Check sheet for the modelled part. Datum: model origin and axes. Units: mm. A direction names the side the tool comes from. Round coordinates to 2 decimals unless told otherwise and drop trailing zeros. Write each loop counter-clockwise with the first axis right and the second up, starting at its lowest first coordinate (ties: lowest second). Pieces come first, ordered by that corner, then holes. Notation, with made-up numbers: (-14.75, -33) -> (43.25, -33) arc R12 cw to (43.25, -14) -> close; hole circle Ø7 at (36, -4). An arc over 180 degrees is marked (long way). Write item = value, one per line.
from build123d import *

# Parameters (mm, degrees)
SKETCH_1_W               = 42
SKETCH_1_H               = 42
SKETCH_1_R               = 1.85
EXTRUDE_1_DEPTH          = 5
FILLET_2_R               = 2
FILLET_3_R               = 2
FILLET_4_R               = 2
FILLET_5_R               = 2
CUT_EXTRUDE_3_DEPTH      = 31.116440693
SKETCH_6_W               = 14
SKETCH_6_H               = 11
CUT_EXTRUDE_4_DEPTH      = 31.116440693
SKETCH_8_R               = 1
CUT_EXTRUDE_6_DEPTH      = 31.116440693
SKETCH_9_R               = 3
CUT_EXTRUDE_7_DEPTH      = 2.7
SKETCH_11_W              = 27.9
SKETCH_11_H              = 28.4
CUT_EXTRUDE_14_DEPTH     = 2.7
CUT_EXTRUDE_15_DEPTH     = 1.5
HOLE_WIZARD_1_AT_2_COUNT = 2
HOLE_WIZARD_1_AT_2_PITCH = 31
HOLE_WIZARD_1_AT_3_COUNT = 2
HOLE_WIZARD_1_AT_3_PITCH = 43.840620434
HOLE_WIZARD_1_AT_4_COUNT = 2
HOLE_WIZARD_1_AT_4_PITCH = 31


with BuildPart() as part:
    # 草图1 → 凸台-拉伸1 (new body)
    with BuildSketch(Plane(origin=(0, 0, 0), x_dir=(1, 0, 0), z_dir=(0, 1, 0))):
        Rectangle(SKETCH_1_W, SKETCH_1_H)
        with Locations(Location((15.5, 15.5, 0), (0, 0, 270))):
            Circle(SKETCH_1_R, mode=Mode.SUBTRACT)
        with Locations(Location((-15.5, 15.5, 0), (0, 0, 270))):
            Circle(SKETCH_1_R, mode=Mode.SUBTRACT)
        with Locations(Location((-15.5, -15.5, 0), (0, 0, 270))):
            Circle(SKETCH_1_R, mode=Mode.SUBTRACT)
        with Locations(Location((15.5, -15.5, 0), (0, 0, 270))):
            Circle(SKETCH_1_R, mode=Mode.SUBTRACT)
    extrude(amount=EXTRUDE_1_DEPTH)

    # 圆角2
    fillet_2_edges = [part.edges().sort_by_distance(p)[0] for p in [
        (-21, 2.5, -21),
    ]]
    fillet(fillet_2_edges, radius=FILLET_2_R)

    # 圆角3
    fillet_3_edges = [part.edges().sort_by_distance(p)[0] for p in [
        (-21, 2.5, 21),
    ]]
    fillet(fillet_3_edges, radius=FILLET_3_R)

    # 圆角4
    fillet_4_edges = [part.edges().sort_by_distance(p)[0] for p in [
        (21, 2.5, 21),
    ]]
    fillet(fillet_4_edges, radius=FILLET_4_R)

    # 圆角5
    fillet_5_edges = [part.edges().sort_by_distance(p)[0] for p in [
        (21, 2.5, -21),
    ]]
    fillet(fillet_5_edges, radius=FILLET_5_R)

    # 草图5 → 切除-拉伸3 (cut, through all)
    with BuildSketch(Plane.XZ):
        Polygon((-15.5, -21), (-10, -15.5), (10, -15.5), (15.5, -21), align=None)
    extrude(amount=-CUT_EXTRUDE_3_DEPTH, mode=Mode.SUBTRACT)

    # 草图6 → 切除-拉伸4 (cut, through all)
    with BuildSketch(Plane.XZ):
        with Locations((-3, 15.5)):
            Rectangle(SKETCH_6_W, SKETCH_6_H)
    extrude(amount=-CUT_EXTRUDE_4_DEPTH, mode=Mode.SUBTRACT)

    # 草图8 → 切除-拉伸6 (cut, through all)
    with BuildSketch(Plane(origin=(0, 5, 0), x_dir=(1, 0, 0), z_dir=(0, 1, 0))):
        with Locations(Location((-14.65, -11, 0), (0, 0, 270))):
            Circle(SKETCH_8_R)
        with Locations(Location((8.65, -11, 0), (0, 0, 270))):
            Circle(SKETCH_8_R)
        with Locations(Location((8.65, 12.8, 0), (0, 0, 270))):
            Circle(SKETCH_8_R)
    extrude(amount=-CUT_EXTRUDE_6_DEPTH, mode=Mode.SUBTRACT)

    # 草图9 → 切除-拉伸7 (cut)
    with BuildSketch(Plane(origin=(0, 5, 0), x_dir=(1, 0, 0), z_dir=(0, 1, 0))):
        with Locations(Location((-15.5, 15.5, 0), (0, 0, 270))):
            Circle(SKETCH_9_R)
        with Locations(Location((15.5, 15.5, 0), (0, 0, 270))):
            Circle(SKETCH_9_R)
        with Locations(Location((15.5, -15.5, 0), (0, 0, 270))):
            Circle(SKETCH_9_R)
        with Locations(Location((-15.5, -15.5, 0), (0, 0, 270))):
            Circle(SKETCH_9_R)
    extrude(amount=-CUT_EXTRUDE_7_DEPTH, mode=Mode.SUBTRACT)

    # 草图11 → 切除-拉伸14 (cut)
    with BuildSketch(Plane(origin=(0, 5, 0), x_dir=(1, 0, 0), z_dir=(0, 1, 0))):
        with Locations((-3, 0.9)):
            Rectangle(SKETCH_11_W, SKETCH_11_H)
    extrude(amount=-CUT_EXTRUDE_14_DEPTH, mode=Mode.SUBTRACT)

    # 草图12 → 切除-拉伸15 (cut)
    with BuildSketch(Plane(origin=(0, 2.3, 0), x_dir=(1, 0, 0), z_dir=(0, 1, 0))):
        Polygon((10.95, -5.871572875), (10.95, 7.671572875), (3.521572875, 15.1), (-9.521572875, 15.1), (-16.95, 7.671572875), (-16.95, -5.871572875), (-9.521572875, -13.3), (3.521572875, -13.3), align=None)
    extrude(amount=-CUT_EXTRUDE_15_DEPTH, mode=Mode.SUBTRACT)

    # 草图14 → 打孔尺寸(%根据十字)槽半沉头木螺钉的类型1 (revolve, cut)
    with BuildSketch(Plane(origin=(15.5, 2.3, 15.5), x_dir=(0, 0, 1), z_dir=(1, 0, 0))):
        Polygon((0, 0), (0, 2.3), (1.8, 2.3), (1.8, 1.5), (3.3, 0), align=None)
    hole_wizard_1 = revolve(axis=Axis((15.5, 8.65, 15.5), (0, -1, 0)), mode=Mode.SUBTRACT)

    # 打孔尺寸(%根据十字)槽半沉头木螺钉的类型1 at 2: 打孔尺寸(%根据十字)槽半沉头木螺钉的类型1 ×2
    with Locations(*[(-i * HOLE_WIZARD_1_AT_2_PITCH, 0, 0) for i in range(1, HOLE_WIZARD_1_AT_2_COUNT)]):
        add(hole_wizard_1, mode=Mode.SUBTRACT)

    # 打孔尺寸(%根据十字)槽半沉头木螺钉的类型1 at 3: 打孔尺寸(%根据十字)槽半沉头木螺钉的类型1 ×2
    with Locations(*[Vector(-0.7071067811865476, 0, -0.7071067811865476) * (i * HOLE_WIZARD_1_AT_3_PITCH) for i in range(1, HOLE_WIZARD_1_AT_3_COUNT)]):
        add(hole_wizard_1, mode=Mode.SUBTRACT)

    # 打孔尺寸(%根据十字)槽半沉头木螺钉的类型1 at 4: 打孔尺寸(%根据十字)槽半沉头木螺钉的类型1 ×2
    with Locations(*[(0, 0, -i * HOLE_WIZARD_1_AT_4_PITCH) for i in range(1, HOLE_WIZARD_1_AT_4_COUNT)]):
        add(hole_wizard_1, mode=Mode.SUBTRACT)


solid = part.part
(1) Sectioned sample at D-D on z = 2.5. Enter the section's corners in (x, y).
Worked answers:
outline = (-21, 0) -> (21, 0) -> (21, 5) -> (10.95, 5) -> (10.95, 0.8) -> (-16.95, 0.8) -> (-16.95, 5) -> (-21, 5) -> close
(2) Sectioned sample at A-A on z = 15.5. Enter the section's corners in (x, y), then the cut area to 3 significant figures.
Worked answers:
outline = (-21, 0) -> (-17.35, 0) -> (-17.35, 0.85) -> (-18.8, 2.3) -> (-18.5, 2.3) -> (-18.5, 5) -> (-21, 5) -> close; (-13.65, 0) -> (-10, 0) -> (-10, 5) -> (-12.5, 5) -> (-12.5, 2.3) -> (-12.2, 2.3) -> (-13.65, 0.85) -> close; (4, 0) -> (13.65, 0) -> (13.65, 0.85) -> (12.2, 2.3) -> (12.5, 2.3) -> (12.5, 5) -> (4, 5) -> close; (17.35, 0) -> (21, 0) -> (21, 5) -> (18.5, 5) -> (18.5, 2.3) -> (18.8, 2.3) -> (17.35, 0.85) -> close
area = 86.4 mm²
(3) Access from +Z, -Z, +X, -X, +Y, -Y to the whole of each face (thin tool, end or side, straight path). Record for faces 1 (the flat face through (17, 2, -21)), 2 (the cylindrical face through (-15.968, 3.669, 18.463)).
Worked answers:
face_1 = -Z, +X, -X, +Y, -Y
face_2 = +Y
(4) Material ranges on L1, parallel to X at y = 2.95, z = 15.5; L2, parallel to X at y = 0.6, z = 15.5; L3, parallel to X at y = 1.35, z = 3, recorded low to high. Write a range as [from, to].
Worked answers:
L1 = [-21, -18.5], [-12.5, -10], [4, 12.5], [18.5, 21]
L2 = [-21, -17.35], [-13.65, -10], [4, 13.65], [17.35, 21]
L3 = [-21, -16.95], [10.95, 21]
(5) Go/stop test with flat-tipped pins: P1, Ø14, axis at x = -4, z = 2, coming from the +Y side; P2, Ø4.5, axis at x = 15.5, z = 15.5, coming from the +Y side; P3, Ø5.5, axis at x = 15.5, z = 15.5, coming from the +Y side. Record where each tip stops, or that it passes through.
Worked answers:
P1 = 0.8
P2 = 1.25
P3 = 1.75
(6) Sectioned sample at B-B on y = 4.25. Enter the section's corners in (x, z), then the cut area to 3 significant figures.
Worked answers:
outline = (-21, -19) arc R2 ccw to (-19, -21) -> (-15.5, -21) -> (-10, -15.5) -> (10, -15.5) -> (15.5, -21) -> (19, -21) arc R2 ccw to (21, -19) -> (21, 19) arc R2 ccw to (19, 21) -> (4, 21) -> (4, 13.3) -> (10.95, 13.3) -> (10.95, -15.1) -> (-12.53, -15.1) arc R3 cw (long way) to (-16.95, -12.87) -> (-16.95, 12.87) arc R3 cw (long way) to (-13.46, 13.3) -> (-10, 13.3) -> (-10, 21) -> (-19, 21) arc R2 ccw to (-21, 19) -> close; hole circle Ø6 at (15.5, -15.5); hole circle Ø6 at (15.5, 15.5)
area = 619 mm²
(7) Sectioned sample at C-C on x = 8.65. Enter the section's corners in (y, z), then the cut area to 3 significant figures.
Worked answers:
outline = (0, -15.5) -> (5, -15.5) -> (5, -15.1) -> (2.3, -15.1) -> (2.3, -13.8) -> (0, -13.8) -> close; (0, -11.8) -> (2.3, -11.8) -> (2.3, -9.97) -> (0.8, -9.97) -> (0.8, 8.17) -> (2.3, 8.17) -> (2.3, 10) -> (0, 10) -> close; (0, 12) -> (2.3, 12) -> (2.3, 13.3) -> (5, 13.3) -> (5, 21) -> (0, 21) -> close
area = 69.4 mm²
(8) Release check for a two-part mould opening along Z. For faces 3 (the flat face through (-13.18, 1.56, -11.44)), 4 (the cylindrical face through (20.4, 2.54, 20.43)), 5 (the flat face through (-21, 2, 0)), 6 (the cylindrical face through (-20.43, 2.54, -20.4)) record: pulls with the +Z half, pulls with the -Z half, needs draft (parallel to the pull), parting line crosses it, or undercut.
Worked answers:
face_3 = undercut
face_4 = pulls with the +Z half
face_5 = needs draft
face_6 = pulls with the -Z half
